Part print with two shaded views. Sizes in mm from the minimum x, y, z corner. A direction names the side the tool comes from. Give positions to 0.01 mm unless a question says otherwise; leave off trailing zeros. Loops run counter-clockwise (first coordinate to the right, second up) from the corner with the lowest first, then second, coordinate; pieces in that order, holes last. Notation, with made-up numbers: (-14.5, -27) -> (4.5, -27) arc R6 cw to (4.5, -23) -> close; hole circle Ø1 at (-27, 17.5). An arc over 180 degrees is marked (long way). One line per question, with ' | ' between items.
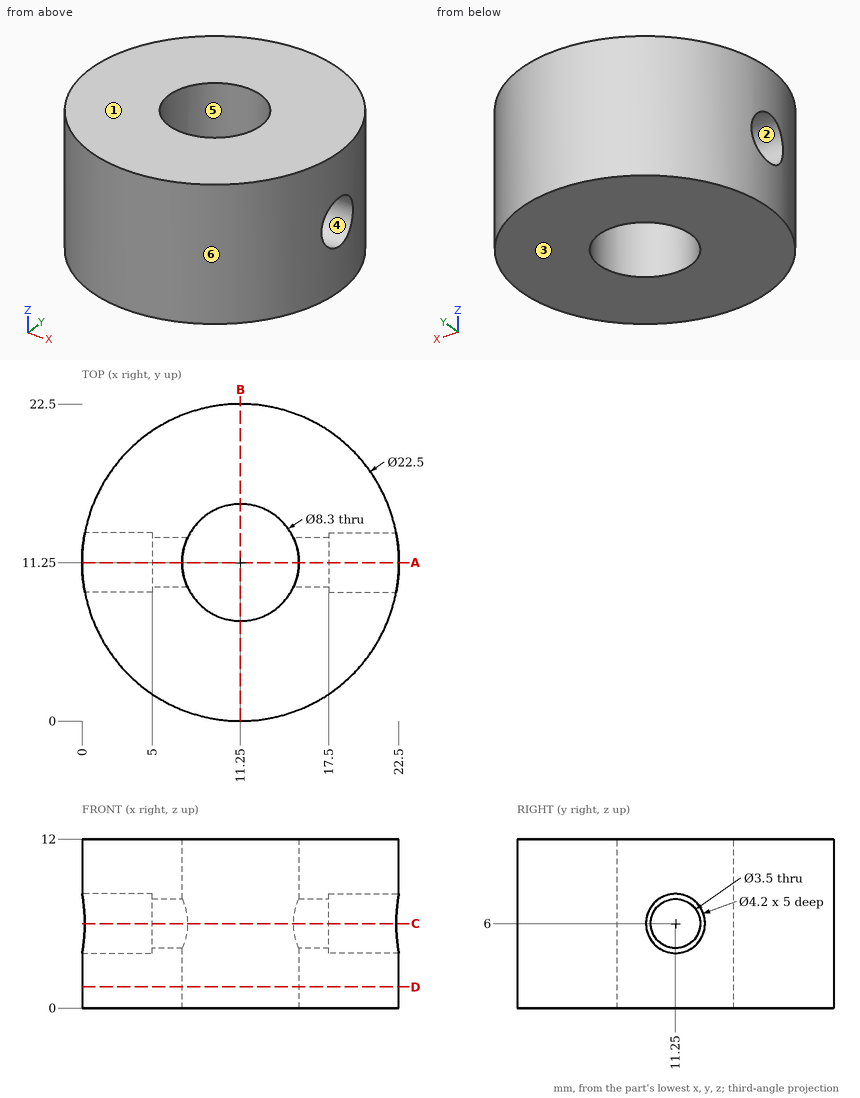
1) Pull direction Y, two halves, no side cores. Call the marked faces 3, 4, 5 and 6: pulls with the +Y half, pulls with the -Y half, needs draft (parallel to the pull), parting line crosses it, or undercut.
Found:
face 3: needs draft | face 4: undercut | face 5: undercut | face 6: parting line crosses it
2) Saw through at C-C (z = 6). Give the cut face in (x, y), and give its area (3 significant figures).
Found:
outline: (0.2, 9.15) arc R11.25 ccw to (22.3, 9.15) -> (17.5, 9.15) -> (17.5, 9.5) -> (15.01, 9.5) arc R4.15 cw to (7.49, 9.5) -> (5, 9.5) -> (5, 9.15) -> close; (0.2, 13.35) -> (5, 13.35) -> (5, 13) -> (7.49, 13) arc R4.15 cw to (15.01, 13) -> (17.5, 13) -> (17.5, 13.35) -> (22.3, 13.35) arc R11.25 ccw to start | area: 286 mm2
3) Saw through at D-D (z = 1.5). Give the cut face in (x, y).
Found:
outline: circle Ø22.5 at (11.25, 11.25); hole circle Ø8.3 at (11.25, 11.25)
4) Tool access for the marked faces 1 and 2: list every direction of +Z, -Z, +X, -X, +Y, -Y with a clear straight run to the whole face (end or side of a thin tool).
Found:
face 1: +Z, +X, -X, +Y, -Y | face 2: -X
5) Saw through at A-A (y = 11.25). Give the cut face in (x, z), and give its area (3 significant figures).
Found:
outline: (0, 0) -> (7.1, 0) -> (7.1, 4.25) -> (5, 4.25) -> (5, 3.9) -> (0, 3.9) -> close; (0, 8.1) -> (5, 8.1) -> (5, 7.75) -> (7.1, 7.75) -> (7.1, 12) -> (0, 12) -> close; (15.4, 0) -> (22.5, 0) -> (22.5, 3.9) -> (17.5, 3.9) -> (17.5, 4.25) -> (15.4, 4.25) -> close; (15.4, 7.75) -> (17.5, 7.75) -> (17.5, 8.1) -> (22.5, 8.1) -> (22.5, 12) -> (15.4, 12) -> close | area: 114 mm2
6) Pin check, flat tips, straight feed: P1, Ø8, axis at x = 13.5, y = 13.5, coming from the -Z side; P2, Ø3, axis at y = 5.5, z = 4, coming from the -X side; P3, Ø5, axis at y = 18, z = 9, coming from the +X side. Stop position of each tip, or through.
Found:
P1: z = 0 | P2: x = 0.83 | P3: x = 21.67
7) Drill centre lines: line 1 (X direction, y = 9.5, z = 7); line 2 (Y direction, x = 6.45, z = 6); line 3 (Y direction, x = 6.9, z = 6). Where is each one in solid material? Low to high.
Found:
line 1: 5 to 7.49, 15.01 to 17.5 | line 2: 1.08 to 9.5, 13 to 21.42 | line 3: 0.88 to 9.5, 13 to 21.62
8) Saw through at B-B (x = 11.25). Give the cut face in (y, z).
Found:
outline: (0, 0) -> (7.1, 0) -> (7.1, 12) -> (0, 12) -> close; (15.4, 0) -> (22.5, 0) -> (22.5, 12) -> (15.4, 12) -> close
